Can you work these out from the model? Positions are in its coordinate system, mm. A direction names the side the tool comes from. Round coordinates to 2 decimals unless told otherwise and drop trailing zeros. Order: outer loops, then holes, each group sorted by start corner. A loop starts at its lowest first (then second) coordinate and runs counter-clockwise, first axis right, second up. Notation, with made-up numbers: (65.25, 17.5) -> (93.25, 17.5) arc R7 cw to (93.25, 30.5) -> close; hole circle Ø8 at (13, 64.25). An arc over 180 degrees is marked (long way). One line per item, written item: value.
```python
from build123d import *

# Parameters (mm, degrees)
CROQUIS1_R              = 16
SALIENTE_EXTRUIR1_DEPTH = 3
CROQUIS2_R              = 8
CROQUIS2_R_2            = 4
SALIENTE_EXTRUIR2_DEPTH = 10
CROQUIS3_R              = 1.95
CORTAR_EXTRUIR1_DEPTH   = 3


with BuildPart() as part:
    # Croquis1 → Saliente-Extruir1 (new body)
    with BuildSketch(Plane.XY):
        Circle(CROQUIS1_R)
    extrude(amount=SALIENTE_EXTRUIR1_DEPTH)

    # Croquis2 → Saliente-Extruir2 (add)
    with BuildSketch(Plane.XY.offset(3)):
        Circle(CROQUIS2_R)
        Circle(CROQUIS2_R_2, mode=Mode.SUBTRACT)
    extrude(amount=SALIENTE_EXTRUIR2_DEPTH)

    # Croquis3 → Cortar-Extruir1 (cut)
    with BuildSketch(Plane.XY.offset(3)):
        with Locations((0, 12)):
            Circle(CROQUIS3_R)
        with Locations((12, 0)):
            Circle(CROQUIS3_R)
        with Locations((0, -12)):
            Circle(CROQUIS3_R)
        with Locations((-12, 0)):
            Circle(CROQUIS3_R)
    extrude(amount=-CORTAR_EXTRUIR1_DEPTH, mode=Mode.SUBTRACT)


solid = part.part
```
Q1. On a 3-axis mill with a long thin cutter (end or side, diameter ignored), from which of +Z, -Z, +X, -X, +Y, -Y can I reach the whole of each face in a straight line? I mean faces 4 (the face through (-0.867, -3.905, 7.93)), 5 (the face through (0, 0, 0)). Say none if no direction works.
Answers below:
face 4: +Z
face 5: -Z, +X, -X, +Y, -Y
Q2. Will these pins go through, and if not, where does the flat tip stop? pin 1 Ø1.5 at (y, z) = (2.5, 10) entering from +X; pin 2 Ø3 at (x, z) = (-6, 8.5) entering from +Y; pin 3 Ø4 at (y, z) = (12.5, 3.5) entering from -X.
Answers below:
pin 1: x = 7.81
pin 2: y = 6.61
pin 3: x = -12.02
Q3. I want a section at D-D on x = -12. List the corners of the cut face in (y, z) for me, plus the area to 3 significant figures.
Answers below:
outline: (-10.58, 0) -> (-1.95, 0) -> (-1.95, 3) -> (-10.58, 3) -> close; (1.95, 0) -> (10.58, 0) -> (10.58, 3) -> (1.95, 3) -> close
area: 51.8 mm^2
Q4. I want a section at C-C on y = 13.5. List the corners of the cut face in (x, z) for me, plus the area to 3 significant figures.
Answers below:
outline: (-8.59, 0) -> (-1.25, 0) -> (-1.25, 3) -> (-8.59, 3) -> close; (1.25, 0) -> (8.59, 0) -> (8.59, 3) -> (1.25, 3) -> close
area: 44.1 mm^2
Q5. Please list where these lines run through material, in increasing order: line 1 along Y through (x, z) = (0, 1.6); line 2 along Y through (x, z) = (0, 5); line 3 along Z through (x, y) = (-8.5, 11.5).
Answers below:
line 1: -16 to -13.95, -10.05 to 10.05, 13.95 to 16
line 2: -8 to -4, 4 to 8
line 3: 0 to 3
Q6. We'd pull the mould along Y, two halves only. Please class faces 1 (the face through (-4, -2, 13)), 2 (the face through (0, 0, 3)), 3 (the face through (-1.73, -7.81, 7.93)): released by +Y, released by -Y, zero draft, split by the parting line, or undercut.
Answers below:
face 1: zero draft
face 2: undercut
face 3: split by the parting line
Q7. I want a section at A-A on x = 0. List the corners of the cut face in (y, z) for me, plus the area to 3 significant figures.
Answers below:
outline: (-16, 0) -> (-13.95, 0) -> (-13.95, 3) -> (-16, 3) -> close; (-10.05, 0) -> (10.05, 0) -> (10.05, 3) -> (8, 3) -> (8, 13) -> (4, 13) -> (4, 3) -> (-4, 3) -> (-4, 13) -> (-8, 13) -> (-8, 3) -> (-10.05, 3) -> close; (13.95, 0) -> (16, 0) -> (16, 3) -> (13.95, 3) -> close
area: 153 mm^2
